from build123d import *

# Parameters (mm, degrees)
CROQUIS1_R              = 1.4
SALIENTE_EXTRUIR1_DEPTH = 1.7
CROQUIS2_W              = 1.7
CROQUIS2_H              = 41.7
SALIENTE_EXTRUIR2_DEPTH = 45.5
REDONDEO1_R             = 20.85
CROQUIS3_R              = 1.55
CORTAR_EXTRUIR1_DEPTH   = 65.26081621


with BuildPart() as part:
    # Croquis1 → Saliente-Extruir1 (new body)
    with BuildSketch(Plane(origin=(0, 0, 0), x_dir=(1, 0, 0), z_dir=(0, 1, 0))):
        with BuildLine():
            Line((-20, -20.85), (17, -20.85))
            ThreePointArc((17, -20.85), (19.121320344, -19.971320344), (20, -17.85))
            Line((20, -17.85), (20, 17.85))
            ThreePointArc((20, 17.85), (19.121320344, 19.971320344), (17, 20.85))
            Line((17, 20.85), (-20, 20.85))
            Line((-20, 20.85), (-20, -20.85))
        make_face()
        with Locations(Location((-12, 15, 0), (0, 0, 270))):
            Circle(CROQUIS1_R, mode=Mode.SUBTRACT)
        with Locations(Location((12, 15, 0), (0, 0, 270))):
            Circle(CROQUIS1_R, mode=Mode.SUBTRACT)
        with Locations(Location((12, -15, 0), (0, 0, 270))):
            Circle(CROQUIS1_R, mode=Mode.SUBTRACT)
        with Locations(Location((-12, -15, 0), (0, 0, 270))):
            Circle(CROQUIS1_R, mode=Mode.SUBTRACT)
    extrude(amount=SALIENTE_EXTRUIR1_DEPTH)

    # Croquis2 → Saliente-Extruir2 (add)
    with BuildSketch(Plane(origin=(0, 1.7, 0), x_dir=(1, 0, 0), z_dir=(0, 1, 0))):
        with Locations((-19.15, 0)):
            Rectangle(CROQUIS2_W, CROQUIS2_H)
    extrude(amount=SALIENTE_EXTRUIR2_DEPTH)

    # Redondeo1
    redondeo1_edges = [part.edges().sort_by_distance(p)[0] for p in [
        (-19.15, 47.2, -20.85),
        (-19.15, 47.2, 20.85),
    ]]
    fillet(redondeo1_edges, radius=REDONDEO1_R - 0.0001)  # a hair under: the kernel refuses the full size

    # Croquis3 → Cortar-Extruir1 (cut, through all)
    with BuildSketch(Plane(origin=(-18.3, 0, 0), x_dir=(0, 0, -1), z_dir=(1, 0, 0))):
        with Locations((15.45, 26.35)):
            Circle(CROQUIS3_R)
        with Locations((7.725, 12.969907512)):
            Circle(CROQUIS3_R)
        with Locations((-7.725, 12.969907512)):
            Circle(CROQUIS3_R)
        with Locations((-15.45, 26.35)):
            Circle(CROQUIS3_R)
        with Locations((-7.725, 39.730092488)):
            Circle(CROQUIS3_R)
        with Locations((7.725, 39.730092488)):
            Circle(CROQUIS3_R)
        with BuildLine():
            Line((6.35, 34.25), (6.35, 20.25))
            ThreePointArc((6.35, 20.25), (0, 13.9), (-6.35, 20.25))
            Line((-6.35, 20.25), (-6.35, 34.25))
            ThreePointArc((-6.35, 34.25), (0, 40.6), (6.35, 34.25))
        make_face()
    extrude(amount=-CORTAR_EXTRUIR1_DEPTH, mode=Mode.SUBTRACT)


solid = part.part
CAD build for the part. Positions are in the model's coordinates, mm. A direction names the side the tool comes from. Round coordinates to 2 decimals unless told otherwise and drop trailing zeros. Write each loop counter-clockwise with the first axis right and the second up, starting at its lowest first coordinate (ties: lowest second). Pieces come first, ordered by that corner, then holes.
(1) Slice it at A-A, the plane x = -12. Write the cut outline in (y, z), and give its area (3 significant figures).
(2) Drop flat-ended pins along their axis: P1, Ø3.5, axis at y = 39.73, z = -7.72, coming from the +X side; P2, Ø12, axis at x = -3, z = -9, coming from the +Y side; P3, Ø1.9, axis at x = -19, y = 28, coming from the -Z side. Give the stop position or say it passes through.
(3) Mould opens along Y. For faces 4 (the face through (1, 1.7, 0)), 5 (the face through (0, 0, 0)), 6 (the face through (-19, 27, 6.35)), 7 (the face through (20, 1, 0)) say: pulls with the +Y half, pulls with the -Y half, needs draft (parallel to the pull), parting line crosses it, or undercut.
(4) Slice it at B-B, the plane z = 15.45. Write the cut outline in (x, y).
(5) Slice it at C-C, the plane y = 36. Write the cut outline in (x, z), and give its area (3 significant figures).
(6) 3-axis set-ups, long thin cutter, end or side, ignore diameter. For faces 1 (the face through (-20, 13, 0)), 2 (the face through (-19, 27, -6.35)), 3 (the face through (-18.3, 14, 5)): which of +Z, -Z, +X, -X, +Y, -Y reach the whole face in a straight line?
(7) Slice it at D-D, the plane x = 7. Write the cut outline in (y, z).
(8) Probe line 1 along Z through (x, y) = (-19, 26); line 2 along X through (y, z) = (2, -7); line 3 along Y through (x, z) = (-1.5, 12). List the from-to ranges inside material, lowest first.
From the geometry:
1. outline: (0, -20.85) - (1.7, -20.85) - (1.7, -16.4) - (0, -16.4) - close; (0, -13.6) - (1.7, -13.6) - (1.7, 13.6) - (0, 13.6) - close; (0, 16.4) - (1.7, 16.4) - (1.7, 20.85) - (0, 20.85) - close
1. area: 61.4 mm2
2. P1: stops at x = -18.3
2. P2: stops at y = 1.7
2. P3: stops at z = -20.84
3. face 4: pulls with the +Y half
3. face 5: pulls with the -Y half
3. face 6: undercut
3. face 7: needs draft
4. outline: (-20, 0) - (-13.33, 0) - (-13.33, 1.7) - (-18.3, 1.7) - (-18.3, 24.8) - (-20, 24.8) - close; (-20, 27.9) - (-18.3, 27.9) - (-18.3, 40.35) - (-20, 40.35) - close; (-10.67, 0) - (10.67, 0) - (10.67, 1.7) - (-10.67, 1.7) - close; (13.33, 0) - (20, 0) - (20, 1.7) - (13.33, 1.7) - close
5. outline: (-20, -18.48) - (-18.3, -18.48) - (-18.3, -6.1) - (-20, -6.1) - close; (-20, 6.1) - (-18.3, 6.1) - (-18.3, 18.48) - (-20, 18.48) - close
5. area: 42.1 mm2
6. face 1: +Z, -Z, -X, +Y, -Y
6. face 2: +X, -X
6. face 3: +Z, -Z, +X, +Y
7. outline: (0, -20.85) - (1.7, -20.85) - (1.7, 20.85) - (0, 20.85) - close
8. line 1: z = -20.85 to -16.96, -13.94 to -6.35, 6.35 to 13.94, 16.96 to 20.85
8. line 2: x = -20 to -18.3
8. line 3: y = 0 to 1.7
